from build123d import *

# Parameters (mm, degrees)
BOSS_EXTRUDE1_DEPTH = 1.6


with BuildPart() as part:
    # Sketch1 → Boss-Extrude1 (new body)
    with BuildSketch(Plane.XY):
        Polygon((-43.3333329, 0), (-129.8399987, 0), (-129.8399987, -1.76), (-216.6666645, -1.76), (-218.4266645, -1.76), (-218.4266645, 0), (-218.4266645, 15.993333333), (-216.6666645, 15.993333333), (-216.6666645, 23.75), (216.6666645, 23.75), (216.6666645, 15.993333333), (218.4266645, 15.993333333), (218.4266645, 0), (218.4266645, -1.76), (216.6666645, -1.76), (130.1599987, -1.76), (130.1599987, 0), (43.6533329, 0), (43.6533329, -1.76), (-43.3333329, -1.76), align=None)
    boss_extrude1 = extrude(amount=BOSS_EXTRUDE1_DEPTH)

    # Mirror1: Boss-Extrude1 across plane
    add(boss_extrude1.mirror(Plane(origin=(216.6666645, 23.75, 1.6), x_dir=(0, 0, 1), z_dir=(0, -1, 0))))


solid = part.part
Design review of the part built by this model. Coordinates are the model's own, in mm. Coordinates: 2 decimals unless noted, no trailing zeros. Write each loop counter-clockwise with the first axis right and the second up, starting at its lowest first coordinate (ties: lowest second). Pieces come first, ordered by that corner, then holes. Notation, with made-up numbers: (49, 3) -> (69, 3) arc R27 cw to (69, 41) -> close; hole circle Ø1 at (-15, -25). An arc over 180 degrees is marked (long way). Write each question's results on one line, items separated by ' | '. Start each with the question number.
(1) For line 1 along X through (y, z) = (23, 0.95); line 2 along Y through (x, z) = (72.5, 1.4), list the stretches that pass through material, from the lowest coordinate up. Write a range as from..to.
(2) Clearance check with flat-ended pins moving along their axes: P1, Ø0.8, axis at x = 83, z = 1, coming from the +Y side; P2, Ø0.5, axis at y = 20, z = 0.5, coming from the -X side. State where each tip first meets the part, or that it passes through.
(3) Take a section at B-B on x = -108.5. Write out the cut boundary in (y, z), and give its area (3 significant figures).
(4) Take a section at A-A on z = 1.05. Write out the cut boundary in (x, y), and give its area (3 significant figures).
Results found:
1) line 1: x = -216.67..216.67 | line 2: y = 0..47.5
2) P1: stops at y = 47.5 | P2: stops at x = -216.67
3) outline: (0, 0) -> (47.5, 0) -> (47.5, 1.6) -> (0, 1.6) -> close | area: 76.0 mm2
4) outline: (-218.43, -1.76) -> (-129.84, -1.76) -> (-129.84, 0) -> (-43.33, 0) -> (-43.33, -1.76) -> (43.65, -1.76) -> (43.65, 0) -> (130.16, 0) -> (130.16, -1.76) -> (218.43, -1.76) -> (218.43, 15.99) -> (216.67, 15.99) -> (216.67, 31.51) -> (218.43, 31.51) -> (218.43, 49.26) -> (130.16, 49.26) -> (130.16, 47.5) -> (43.65, 47.5) -> (43.65, 49.26) -> (-43.33, 49.26) -> (-43.33, 47.5) -> (-129.84, 47.5) -> (-129.84, 49.26) -> (-218.43, 49.26) -> (-218.43, 31.51) -> (-216.67, 31.51) -> (-216.67, 15.99) -> (-218.43, 15.99) -> close | area: 21,600 mm2
